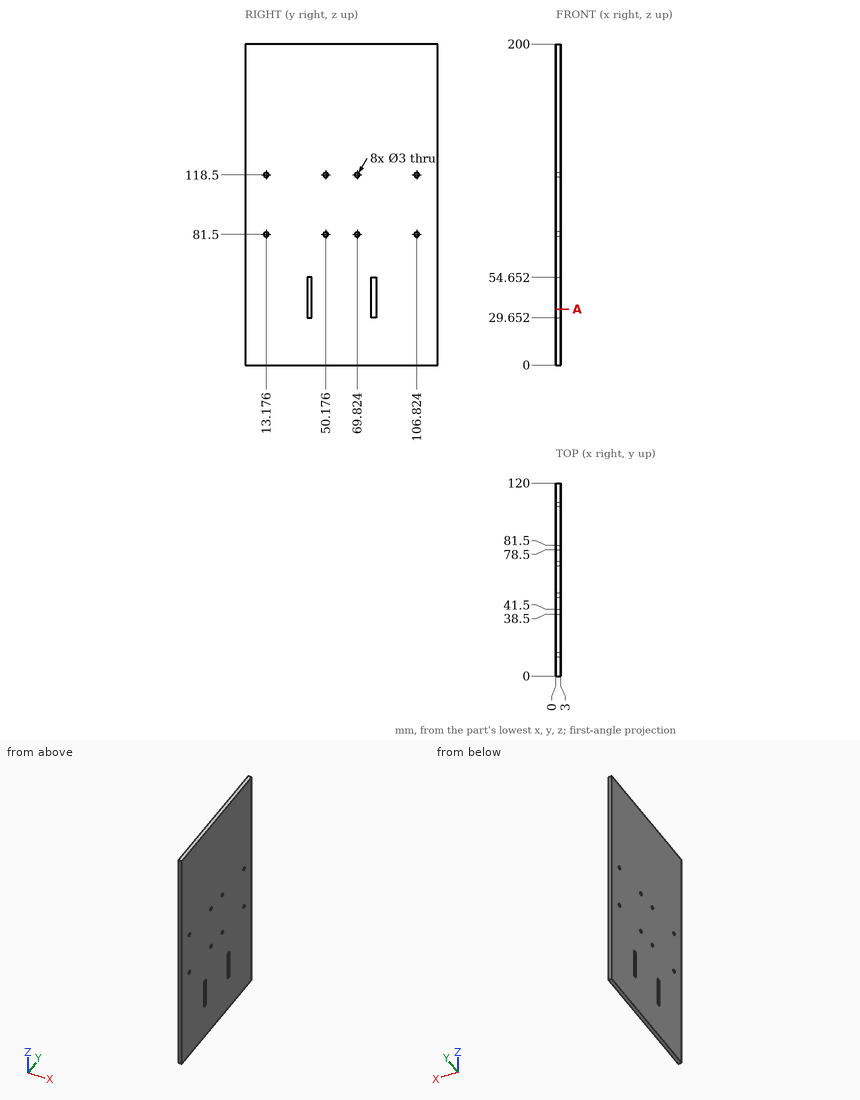
Could you check a few things on this drawing? It's one solid part, dimensions in mm from its lowest x, y, z. Coordinates: 2 decimals unless noted, no trailing zeros. Order: outer loops, then holes, each group sorted by start corner. A loop starts at its lowest first (then second) coordinate and runs counter-clockwise, first axis right, second up. Notation, with made-up numbers: (-19, -13) -> (-10, -13) arc R20 cw to (-10, 22) -> close; hole circle Ø8 at (-22.5, 67). An arc over 180 degrees is marked (long way). One line per item, written item: value. Start each with the question number.
1) If I drill on L1, parallel to Y at x = 1.45, z = 81.5 (1 decimal); L2, parallel to Y at x = 2.1, z = 45.5; L3, parallel to Z at x = 1, y = 50, over which ranges is the centre line in solid material (lowest first)? Write a range as [from, to].
2) I'm going to push flat-ended pins straight in: pin 1 (5 mm diameter, centred on y = 50.18, z = 81.5, fed in from -X); pin 2 (2.5 mm diameter, centred on y = 106.82, z = 81.5, fed in from +X). Where does each tip first touch, or does it pass through?
3) Imagine slicing it at A-A on z = 35. List the corners of the cut face in (x, y) for me.
Answer list:
1. L1: y = [0, 11.7], [14.7, 48.7], [51.7, 68.3], [71.3, 105.3], [108.3, 120]
1. L2: y = [0, 38.5], [41.5, 78.5], [81.5, 120]
1. L3: z = [0, 80.01], [82.99, 117.01], [119.99, 200]
2. pin 1: stops at x = 0
2. pin 2: passes through
3. outline: (0, 0) -> (3, 0) -> (3, 38.5) -> (0, 38.5) -> close; (0, 41.5) -> (3, 41.5) -> (3, 78.5) -> (0, 78.5) -> close; (0, 81.5) -> (3, 81.5) -> (3, 120) -> (0, 120) -> close
